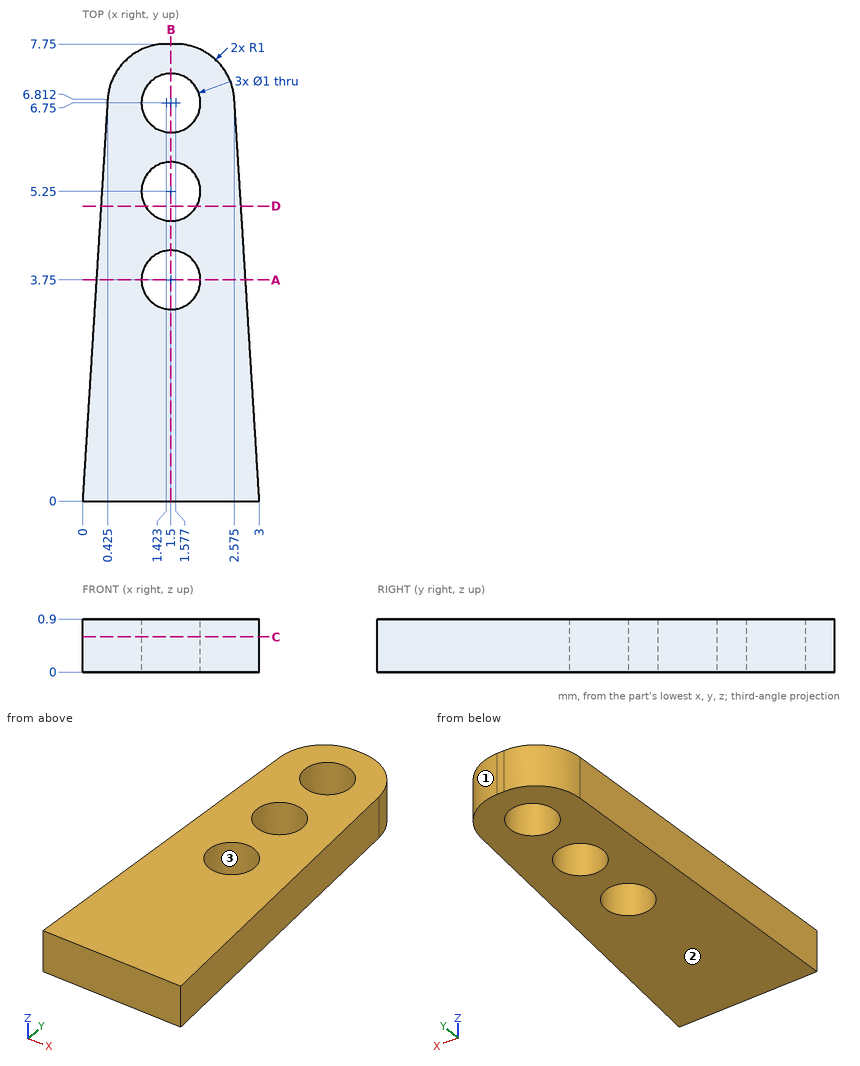
Answer from the drawing. Dimensions are ordinates in mm from the lowest x, y and z of the part. Round coordinates to 2 decimals unless told otherwise and drop trailing zeros. Loops run counter-clockwise (first coordinate to the right, second up) from the corner with the lowest first, then second, coordinate; pieces in that order, holes last.
Q1. Section A-A on y = 3.75 is taken. Write down the section's boundary in (x, z).
Q2. Consider probe 1 along Y at (x, z) = (1.5, 0.6); probe 2 along Y at (x, z) = (1.25, 0.2) (1 decimal); probe 3 along X at (y, z) = (3.5, 0.6). Determine where each line is inside the solid, lowest interval first.
Q3. This flat-tipped pin is pushed along its axis until it touches: pin 1 (1.5 mm diameter, centred on x = 1, y = 2.5, fed in from -Z). Where does it stop, or does it pass through?
Q4. Determine the mould class of the marked faces 1, 2 and 3 for opening direction Y: released by +Y, released by -Y, zero draft, split by the parting line, or undercut.
Q5. Section C-C on z = 0.6 is taken. Give the number of separate pieces and of enclosed holes in the cut face, and give its area (3 significant figures).
Q6. Section D-D on y = 5 is taken. Write down the section's boundary in (x, z).
Q7. Section B-B on x = 1.5 is taken. Write down the section's boundary in (y, z).
Output:
1. outline: (0.23, 0) - (1, 0) - (1, 0.9) - (0.23, 0.9) - close; (2, 0) - (2.77, 0) - (2.77, 0.9) - (2, 0.9) - close
2. probe 1: y = 0 to 3.25, 4.25 to 4.75, 5.75 to 6.25, 7.25 to 7.75
2. probe 2: y = 0 to 3.3, 4.2 to 4.8, 5.7 to 6.3, 7.2 to 7.7
2. probe 3: x = 0.22 to 1.07, 1.93 to 2.78
3. pin 1: stops at z = 0
4. face 1: released by +Y
4. face 2: zero draft
4. face 3: undercut
5. separate pieces: 1
5. enclosed holes: 3
5. area: 16.8 mm2
6. outline: (0.31, 0) - (1.07, 0) - (1.07, 0.9) - (0.31, 0.9) - close; (1.93, 0) - (2.69, 0) - (2.69, 0.9) - (1.93, 0.9) - close
7. outline: (0, 0) - (3.25, 0) - (3.25, 0.9) - (0, 0.9) - close; (4.25, 0) - (4.75, 0) - (4.75, 0.9) - (4.25, 0.9) - close; (5.75, 0) - (6.25, 0) - (6.25, 0.9) - (5.75, 0.9) - close; (7.25, 0) - (7.75, 0) - (7.75, 0.9) - (7.25, 0.9) - close
